Check sheet for the modelled part. Datum: model origin and axes. Units: mm. A direction names the side the tool comes from. Give positions to 0.01 mm unless a question says otherwise; leave off trailing zeros. Write each loop counter-clockwise with the first axis right and the second up, starting at its lowest first coordinate (ties: lowest second). Pieces come first, ordered by that corner, then holes. Notation, with made-up numbers: M 74.5,86 L 93.5,86 A12 cw 93.5,103 Z; hole C 21,-16.75 d8. An arc over 180 degrees is marked long. Use CSV: the item, a comma, the result in double quotes. Start each with the question number.
1. Cross-section at B-B, the plane x = 1508.5. Enter the section's corners in (y, z).
2. Mould release check, pull along X, two halves, no side actions. Record for faces 1 (the face through (308.102, -456, 642)), 2 (the face through (327, -495, 0)), 3 (the face through (1806.702, -456, 603)): +X half, -X half, draft (parallel to the pull), parting line (faces both ways), or undercut.
3. Depth check by flat-ended pin: P1, Ø21, axis at y = -277, z = 1062.5, coming from the +X side (3 decimals); P2, Ø14, axis at y = -275, z = 1082.5, coming from the -X side; P3, Ø11.5, axis at x = 1824.5, z = 552.5, coming from the +Y side. Enter the tip coordinate at first touch or a pass-through.
4. Cross-section at D-D, the plane y = -524. Enter the section's corners in (x, z) (3 decimals).
5. Access from +Z, -Z, +X, -X, +Y, -Y to the whole of each face (thin tool, end or side, straight path). Record for faces 4 (the face through (1066, -495, 1016)), 5 (the face through (1825, -444.5, 485)), 6 (the face through (1073, -546.1, 1032)), 7 (the face through (1066, -444.5, 1035)), 8 (the face through (1844.802, -456, 642)).
6. Cross-section at C-C, the plane y = -359. Enter the section's corners in (x, z) (3 decimals).
7. Scan lines: line 1 (X direction, y = -412.5, z = 1022); line 2 (Z direction, x = 1382, y = -286); line 3 (Z direction, x = 790, y = -486.5). Record each from-to range of solid material in increasing order.
8. Cross-section at A-A, the plane z = 139.5. Enter the section's corners in (x, y).
from build123d import *

# Parameters (mm, degrees)
BOX011_W     = 38.1
BOX011_H     = 546.1
BOX011_DEPTH = 69.85
BOX010_W     = 38.1
BOX010_H     = 101.6
BOX010_DEPTH = 1054.1
BOX013_W     = 38.1
BOX013_H     = 546.1
BOX013_DEPTH = 69.85
BOX012_W     = 38.1
BOX012_H     = 101.6
BOX012_DEPTH = 1054.1
BOX014_W     = 1460.5
BOX014_H     = 101.6
BOX014_DEPTH = 38.1
BOX009_W     = 1803.4
BOX009_H     = 609.6
BOX009_DEPTH = 12.7
BOX008_W     = 1828.8
BOX008_H     = 609.6
BOX008_DEPTH = 19.05


with BuildPart() as cube005:
    # Box011 → Box011 (new body)
    with BuildSketch(Plane(origin=(308.102, -546.1, 984.25), x_dir=(1, 0, 0), z_dir=(0, 0, 1))):
        with Locations((19.05, 273.05)):
            Rectangle(BOX011_W, BOX011_H)
    extrude(amount=BOX011_DEPTH)


with BuildPart() as tableleg:
    # Box010 → Box010 (new body)
    with BuildSketch(Plane(origin=(308.102, -546.1, 0), x_dir=(1, 0, 0), z_dir=(0, 0, 1))):
        with Locations((19.05, 50.8)):
            Rectangle(BOX010_W, BOX010_H)
    extrude(amount=BOX010_DEPTH)

    # Fusion002: union Cube005
    add(cube005.part)


with BuildPart() as cube007:
    # Box013 → Box013 (new body)
    with BuildSketch(Plane(origin=(1806.702, -546.1, 984.25), x_dir=(1, 0, 0), z_dir=(0, 0, 1))):
        with Locations((19.05, 273.05)):
            Rectangle(BOX013_W, BOX013_H)
    extrude(amount=BOX013_DEPTH)


with BuildPart() as tableleg2:
    # Box012 → Box012 (new body)
    with BuildSketch(Plane(origin=(1806.702, -546.1, 0), x_dir=(1, 0, 0), z_dir=(0, 0, 1))):
        with Locations((19.05, 50.8)):
            Rectangle(BOX012_W, BOX012_H)
    extrude(amount=BOX012_DEPTH)

    # Fusion003: union Cube007
    add(cube007.part)


with BuildPart() as cube008:
    # Box014 → Box014 (new body)
    with BuildSketch(Plane(origin=(346.202, -546.1, 1016), x_dir=(1, 0, 0), z_dir=(0, 0, 1))):
        with Locations((730.25, 50.8)):
            Rectangle(BOX014_W, BOX014_H)
    extrude(amount=BOX014_DEPTH)


with BuildPart() as cube003:
    # Box009 → Box009 (new body)
    with BuildSketch(Plane(origin=(168.402, -609.6, 1073.15), x_dir=(1, 0, 0), z_dir=(0, 0, 1))):
        with Locations((901.7, 304.8)):
            Rectangle(BOX009_W, BOX009_H)
    extrude(amount=BOX009_DEPTH)


with BuildPart() as table:
    # Box008 → Box008 (new body)
    with BuildSketch(Plane(origin=(142.875, -609.6, 1054.1), x_dir=(1, 0, 0), z_dir=(0, 0, 1))):
        with Locations((914.4, 304.8)):
            Rectangle(BOX008_W, BOX008_H)
    extrude(amount=BOX008_DEPTH)

    # Fusion: union Cube003
    add(cube003.part)

    # Fusion004: union TableLeg, TableLeg2, Cube008
    add(tableleg.part)
    add(tableleg2.part)
    add(cube008.part)


solid = table.part
Worked answers:
1,outline,"M -609.6,1054.1 L -546.1,1054.1 L -546.1,1016 L -444.5,1016 L -444.5,1054.1 L 0,1054.1 L 0,1085.85 L -609.6,1085.85 Z"
2,face 1,"-X half"
2,face 2,"draft"
2,face 3,"undercut"
3,P1,"stops at x = 1971.675"
3,P2,"stops at x = 168.4"
3,P3,"stops at y = -444.5"
4,outline,"M 142.875,1054.1 L 308.102,1054.1 L 308.102,0 L 346.202,0 L 346.202,1016 L 1806.702,1016 L 1806.702,0 L 1844.802,0 L 1844.802,1054.1 L 1971.675,1054.1 L 1971.675,1073.15 L 1971.802,1073.15 L 1971.802,1085.85 L 168.402,1085.85 L 168.402,1073.15 L 142.875,1073.15 Z"
5,face 4,"-Z, +Y, -Y"
5,face 5,"-Z, +X, -X, +Y"
5,face 6,"-Z, +X, -X, -Y"
5,face 7,"-Z, +Y"
5,face 8,"-Z, +X, +Y, -Y"
6,outline,"M 142.875,1054.1 L 308.102,1054.1 L 308.102,984.25 L 346.202,984.25 L 346.202,1054.1 L 1806.702,1054.1 L 1806.702,984.25 L 1844.802,984.25 L 1844.802,1054.1 L 1971.675,1054.1 L 1971.675,1073.15 L 1971.802,1073.15 L 1971.802,1085.85 L 168.402,1085.85 L 168.402,1073.15 L 142.875,1073.15 Z"
7,line 1,"x = 308.1 to 346.2, 1806.7 to 1844.8"
7,line 2,"z = 1054.1 to 1085.85"
7,line 3,"z = 1016 to 1085.85"
8,outline,"M 308.1,-546.1 L 346.2,-546.1 L 346.2,-444.5 L 308.1,-444.5 Z; M 1806.7,-546.1 L 1844.8,-546.1 L 1844.8,-444.5 L 1806.7,-444.5 Z"
